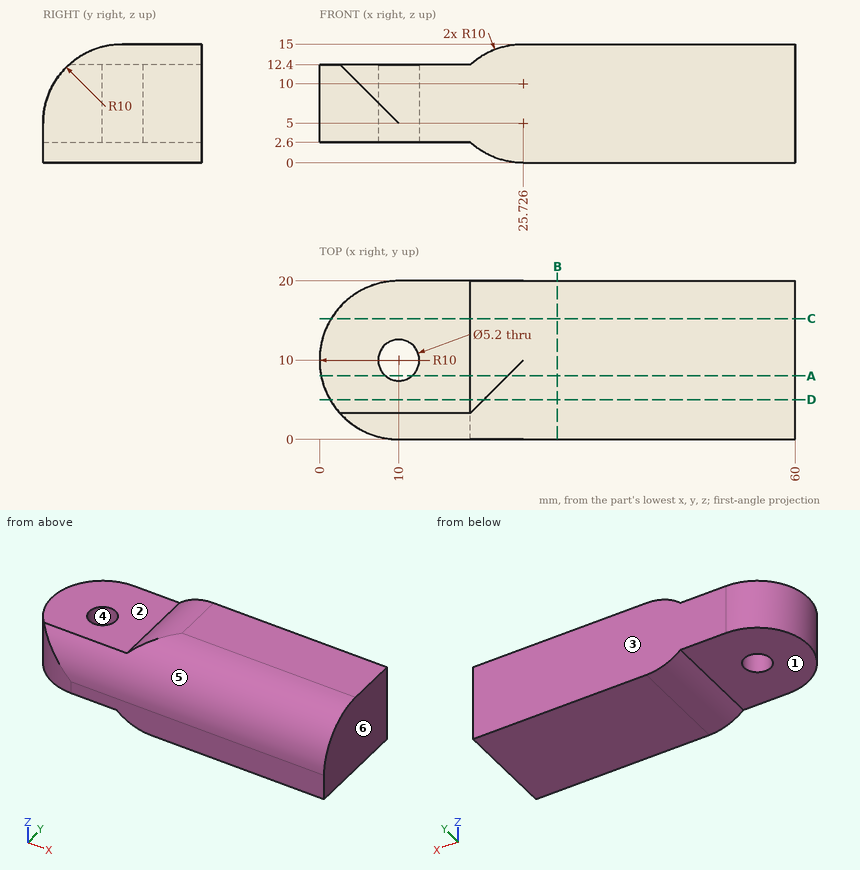
Answer from the drawing. Dimensions are ordinates in mm from the lowest x, y and z of the part. A direction names the side the tool comes from. Give positions to 0.01 mm unless a question says otherwise; leave off trailing zeros. Loops run counter-clockwise (first coordinate to the right, second up) from the corner with the lowest first, then second, coordinate; pieces in that order, holes last.
Item 1: Find the intervals of material crossed by line 1 along X through (y, z) = (10.25, 4.5); line 2 along Y through (x, z) = (10, 9) (3 decimals); line 3 along Z through (x, y) = (19, 6.75), in increasing order.
Derived:
line 1: x = 0 to 7.41, 12.59 to 60
line 2: y = 0.835 to 7.4, 12.6 to 20
line 3: z = 2.6 to 12.4
Item 2: Determine the mould class of the marked faces 4, 5 and 6 for opening direction Y: +Y half, -Y half, draft (parallel to the pull), parting line (faces both ways), or undercut.
Derived:
face 4: undercut
face 5: -Y half
face 6: draft
Item 3: A cutting plane is placed at C-C (y = 15.25). Give the vertices of the cut face in (x, z).
Derived:
outline: (1.49, 2.6) - (19, 2.6) arc R10 ccw to (25.73, 0) - (60, 0) - (60, 15) - (25.73, 15) arc R10 ccw to (19, 12.4) - (1.49, 12.4) - close
Item 4: Each of these flat-tipped pins is pushed along its axis until it touches: pin 1 Ø1.5 at (x, z) = (12.5, 13.5) entering from +Y; pin 2 Ø8.5 at (x, y) = (7, 10) entering from +Z; pin 3 Ø8 at (y, z) = (16.5, 11) entering from -X; pin 4 Ø6 at (x, z) = (30, 8.5) entering from -Y. Where does it stop, or does it pass through?
Derived:
pin 1: passes through
pin 2: stops at z = 12.4
pin 3: stops at x = 0.32
pin 4: stops at y = 0.01
Item 5: A cutting plane is placed at A-A (y = 8). Give the vertices of the cut face in (x, z), then the cut area to 4 significant figures.
Derived:
outline: (0.2, 2.6) - (8.34, 2.6) - (8.34, 12.4) - (0.2, 12.4) - close; (11.66, 2.6) - (19, 2.6) arc R10 ccw to (25.73, 0) - (60, 0) - (60, 14.8) - (23.73, 14.8) arc R10 ccw to (19, 12.4) - (11.66, 12.4) - close
area: 748.5 mm2
Item 6: A cutting plane is placed at B-B (x = 30). Give the vertices of the cut face in (y, z), then the cut area to 3 significant figures.
Derived:
outline: (0, 0) - (20, 0) - (20, 15) - (10, 15) arc R10 ccw to (0, 5) - close
area: 279 mm2
Item 7: A tool of negligible diameter and unlimited length cuts with its end or side. For the marked faces 1, 2 and 3, from which of +Z, -Z, +X, -X, +Y, -Y can it reach the whole face along a straight path? Write none if from no direction.
Derived:
face 1: -Z, -X, +Y, -Y
face 2: +Z, -X, +Y, -Y
face 3: +Z, -Z, +X, -X, +Y
Item 8: A cutting plane is placed at D-D (y = 5). Give the vertices of the cut face in (x, z).
Derived:
outline: (1.34, 2.6) - (19, 2.6) arc R10 ccw to (25.73, 0) - (60, 0) - (60, 13.66) - (20.73, 13.66) arc R10 ccw to (19, 12.4) - (1.34, 12.4) - close
